Here's how the part is built. I have some questions about the finished solid (model axes, mm). Face numbers are marked on the shaded views. A direction names the side the tool comes from. Round coordinates to 2 decimals unless told otherwise and drop trailing zeros. Order: outer loops, then holes, each group sorted by start corner. A loop starts at its lowest first (then second) coordinate and runs counter-clockwise, first axis right, second up. Notation, with made-up numbers: (-32.75, 15.5) - (-12.75, 15.5) arc R14 ccw to (-12.75, 23.5) - close; hole circle Ø8 at (-15, 3). An arc over 180 degrees is marked (long way). Answer as a JSON object with one key per item and string values.
Autodesk Inventor part; units mm, degrees
sketch "Эскиз1" plane through (0, 0, 0) normal (0, 0, 1) x (1, 0, 0)
  line L0 (-11.0294, 43.3824) -> (-11.0294, -6.6176)
  line L1 (-11.0294, -6.6176) -> (18.9706, -6.6176)
  line L2 (18.9706, -6.6176) -> (-11.0294, 43.3824)
  line L3 (-11.0294, -6.6176) -> (11.0294, 6.6176) construction
  line L4 (-6.0294, -6.6176) -> (0.9706, -6.6176)
  line L5 (0.9706, -6.6176) -> (0.9706, -10.6176)
  line L6 (0.9706, -10.6176) -> (-6.0294, -10.6176)
  line L7 (-6.0294, -10.6176) -> (-6.0294, -6.6176)
  line L8 (6.9706, -6.6176) -> (13.9706, -6.6176)
  line L9 (13.9706, -6.6176) -> (13.9706, -10.6176)
  line L10 (13.9706, -10.6176) -> (6.9706, -10.6176)
  line L11 (6.9706, -10.6176) -> (6.9706, -6.6176)
  line L12 (-11.0294, 28.3824) -> (-15.0294, 28.3824)
  line L13 (-15.0294, 28.3824) -> (-15.0294, 18.3824)
  line L14 (-15.0294, 18.3824) -> (-11.0294, 18.3824)
  line L15 (-11.0294, 18.3824) -> (-11.0294, 28.3824)
  line L16 (-11.0294, -1.6176) -> (-15.0294, -1.6176)
  line L17 (-15.0294, -1.6176) -> (-15.0294, 8.3824)
  line L18 (-15.0294, 8.3824) -> (-11.0294, 8.3824)
  line L19 (-11.0294, 8.3824) -> (-11.0294, -1.6176)
  point P0 (0, 0)
  point P1 (0, 0)
  point P2 (-11.0294, 8.3824)
  point P3 (0.9706, -6.6176)
  dimension "d0" = 30
  dimension "d1" = 50
  dimension "d2" = 10
  dimension "d3" = 15
  dimension "d4" = 4
  dimension "d5" = 5
  dimension "d6" = 5
  dimension "d7" = 7
  dimension "d8" = 5
extrude "Выдавливание1" add sketch "Эскиз1" along normal mid plane 4
sketch "Эскиз2" plane through (0, 0, 2) normal (0, 0, 1) x (1, 0, 0)
  line L0 (-11.0294, 18.3824) -> (-11.0294, 8.3824)
  line L1 (-11.0294, 14.8324) -> (-1.0294, 14.8324)
  line L2 (-1.0294, 14.8324) -> (-1.0294, 11.9324)
  line L3 (-1.0294, 11.9324) -> (-11.0294, 11.9324)
  line L4 (-11.0294, 11.9324) -> (-11.0294, 14.8324)
  line L5 (0.9706, -6.6176) -> (6.9706, -6.6176)
  line L6 (2.5206, -6.6176) -> (5.4206, -6.6176)
  line L7 (5.4206, -6.6176) -> (5.4206, 3.3824)
  line L8 (5.4206, 3.3824) -> (2.5206, 3.3824)
  line L9 (2.5206, 3.3824) -> (2.5206, -6.6176)
  line L10 (-6.0294, 16.2824) -> (-3.7294, 16.2824)
  line L11 (-3.7294, 16.2824) -> (-3.7294, 10.4824)
  line L12 (-3.7294, 10.4824) -> (-6.0294, 10.4824)
  line L13 (-6.0294, 10.4824) -> (-6.0294, 16.2824)
  line L14 (1.0706, 0.6824) -> (6.8706, 0.6824)
  line L15 (6.8706, 0.6824) -> (6.8706, -1.6176)
  line L16 (6.8706, -1.6176) -> (1.0706, -1.6176)
  line L17 (1.0706, -1.6176) -> (1.0706, 0.6824)
  line L18 (-11.0294, 13.3824) -> (-1.0294, 13.3824) construction
  line L19 (3.9706, 3.3824) -> (3.9706, -6.6176) construction
  point P0 (0, 0)
  point P1 (-3.7294, 13.3824)
  point P2 (3.9706, 0.6824)
  point P3 (-6.0294, 14.8324)
  point P4 (-11.0294, 11.9324)
  point P5 (-6.0294, 11.9324)
  point P6 (-3.7294, 11.9324)
  point P7 (-3.7294, 14.8324)
  point P8 (2.5206, -1.6176)
  point P9 (5.4206, -1.6176)
  point P10 (5.4206, 0.6824)
  point P11 (2.5206, 0.6824)
  dimension "d11" = 2.9
  dimension "d12" = 10
  dimension "d13" = 2.3
  dimension "d14" = 5.8
  dimension "d15" = 5
  dimension "d16" = 5
extrude "Выдавливание2" cut sketch "Эскиз2" against normal up to next
properties part number "Рёбра_жёсткости"
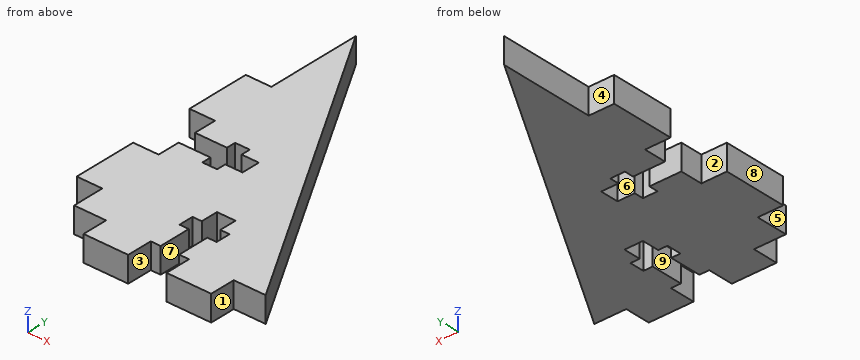
1. For the marked faces 1, 2, 3, 4 and 5, which set-ups out of +Z, -Z, +X, -X, +Y, -Y let a thin tool reach every point of the face, with its end or its side?
Responses:
{"face 1": "+Z, -Z, +X, -Y", "face 2": "+Z, -Z, -X", "face 3": "+Z, -Z, -Y", "face 4": "+Z, -Z, -X, +Y", "face 5": "+Z, -Z, -X, -Y"}
2. Imagine slicing it at B-B (y = 2). List the corners of the cut face in (x, z) for me.
Responses:
{"outline": "(-15.03, -2) - (2.52, -2) - (2.52, 2) - (-15.03, 2) - close; (5.42, -2) - (13.8, -2) - (13.8, 2) - (5.42, 2) - close"}
3. If I drill on L1, parallel to X at y = -7, z = -0.15; L2, parallel to Y at x = -10, z = 1.75; L3, parallel to Y at x = -1.5, z = -0.6, over which ranges is the centre line in solid material (lowest first)? Write a range as [from, to].
Responses:
{"L1": "[-6.03, 0.97], [6.97, 13.97]", "L2": "[-6.62, 11.93], [14.83, 41.67]", "L3": "[-10.62, 11.93], [14.83, 27.5]"}
4. For P1, Ø1.2, axis at x = -8.5, z = 1, coming from the -Y side; P2, Ø1.8, axis at y = -1, z = 1, coming from the +X side; P3, Ø0.9, axis at y = 13, z = 0.5, coming from the -X side, each with a flat end and sliding along its axis, tell me the tip position at first contact or that it passes through.
Responses:
{"P1": "y = -6.62", "P2": "x = 16.14", "P3": "x = -1.03"}
5. Thinking about a two-plate mould opening in X: for the marked faces 6, 7, 8 and 9, which applies, pulls with the +X half, pulls with the -X half, needs draft (parallel to the pull), parting line crosses it, or undercut?
Responses:
{"face 6": "needs draft", "face 7": "undercut", "face 8": "pulls with the -X half", "face 9": "undercut"}
6. Imagine slicing it at A-A (x = -4.5). List the corners of the cut face in (y, z) for me.
Responses:
{"outline": "(-10.62, -2) - (10.48, -2) - (10.48, 2) - (-10.62, 2) - close; (16.28, -2) - (32.5, -2) - (32.5, 2) - (16.28, 2) - close"}
7. Imagine slicing it at D-D (x = 12). List the corners of the cut face in (y, z) for me, plus the area to 3 significant figures.
Responses:
{"outline": "(-10.62, -2) - (5, -2) - (5, 2) - (-10.62, 2) - close", "area": "62.5 mm2"}
8. Imagine slicing it at C-C (y = 35). List the corners of the cut face in (x, z) for me.
Responses:
{"outline": "(-11.03, -2) - (-6, -2) - (-6, 2) - (-11.03, 2) - close"}
